Build history of the part. All positions in model axes, mm. Face numbers are marked on the shaded views. A direction names the side the tool comes from. Give positions to 0.01 mm unless a question says otherwise; leave off trailing zeros. Loops run counter-clockwise (first coordinate to the right, second up) from the corner with the lowest first, then second, coordinate; pieces in that order, holes last. Notation, with made-up numbers: M 65.25,50.25 L 72.25,50.25 A34 cw 72.25,89.25 Z; hole C -29.75,6 d4. An arc over 180 degrees is marked long. Put each result on its own line as item: value.
```python
from build123d import *

# Parameters (mm, degrees)
F1_DEPTH      = 19.05
F2_R          = 8.200531
F3_DEPTH      = 38.1
F3_DEPTH_BACK = 25.4
F5_DEPTH      = 38.1


with BuildPart() as f1:
    # F0 (on Front) → F1 (new body, symmetric)
    with BuildSketch(Plane.XZ):
        with BuildLine():
            Line((-32.141831, 33.15654), (-26.644221, 0))
            Line((-26.644221, 0), (-32.141831, -48.038937))
            Line((-32.141831, -48.038937), (-37.479226, -82.203552))
            Line((-37.479226, -82.203552), (-48.503112, -88.604517))
            Line((-48.503112, -88.604517), (-48.503112, -100.208476))
            Line((-48.503112, -100.208476), (-13.84278, -100.208476))
            Line((-13.84278, -100.208476), (0, -20.61474))
            Line((0, -20.61474), (0, 124.924347))
            ThreePointArc((0, 124.924347), (-20.562864, 109.037436), (-6.345349, 87.28686))
            Line((-6.345349, 87.28686), (-18.186359, 69.102459))
            Line((-18.186359, 69.102459), (-43.982837, 61.913271))
            Line((-43.982837, 61.913271), (-71.473219, 31.58654))
            Line((-71.473219, 31.58654), (-64.171686, 6.32793))
            Line((-64.171686, 6.32793), (-53.286485, 9.474526))
            Line((-53.286485, 9.474526), (-57.54343, 24.200819))
            Line((-57.54343, 24.200819), (-43.137055, 42.037293))
            Line((-43.137055, 42.037293), (-32.141831, 33.15654))
        make_face()
        with BuildLine():
            Line((0, 124.924347), (0, -20.61474))
            Line((0, -20.61474), (13.84278, -100.208476))
            Line((13.84278, -100.208476), (48.503112, -100.208476))
            Line((48.503112, -100.208476), (48.503112, -88.604517))
            Line((48.503112, -88.604517), (37.479226, -82.203552))
            Line((37.479226, -82.203552), (32.141831, -48.038937))
            Line((32.141831, -48.038937), (26.644221, 0))
            Line((26.644221, 0), (32.141831, 33.15654))
            Line((32.141831, 33.15654), (43.137055, 42.037293))
            Line((43.137055, 42.037293), (57.54343, 24.200819))
            Line((57.54343, 24.200819), (53.286485, 9.474526))
            Line((53.286485, 9.474526), (64.171686, 6.32793))
            Line((64.171686, 6.32793), (71.473219, 31.58654))
            Line((71.473219, 31.58654), (43.982837, 61.913271))
            Line((43.982837, 61.913271), (18.186359, 69.102459))
            Line((18.186359, 69.102459), (6.345349, 87.28686))
            ThreePointArc((6.345349, 87.28686), (20.562864, 109.037436), (0, 124.924347))
        make_face()
    extrude(amount=F1_DEPTH, both=True)

    # F2 (on face) → F3 (cut, two sides)
    with BuildSketch(Plane.XZ.offset(19.05)) as f3_sk:
        with Locations((-10.217502, 107.796535)):
            Circle(F2_R)
        with Locations((10.217502, 107.796535)):
            Circle(F2_R)
    extrude(amount=-F3_DEPTH, mode=Mode.SUBTRACT)
    extrude(f3_sk.sketch, amount=-F3_DEPTH_BACK, mode=Mode.SUBTRACT)

    # F4 (on face) → F5 (join, through all)
    with BuildSketch(Plane(origin=(0, 19.05, 0), x_dir=(-1, 0, 0), z_dir=(0, 1, 0))):
        with BuildLine():
            ThreePointArc((-6.158323, 124.468817), (-8.54694, 126.271077), (-9.095944, 129.212543))
            ThreePointArc((-9.095944, 129.212543), (-10.942716, 126.29527), (-10.440769, 122.879263))
            ThreePointArc((-10.440769, 122.879263), (-8.347127, 123.802228), (-6.158323, 124.468817))
        make_face()
        with BuildLine():
            ThreePointArc((-16.136752, 118.410561), (-15.235, 119.378746), (-14.268527, 120.282334))
            ThreePointArc((-14.268527, 120.282334), (-15.496071, 121.489871), (-15.748994, 123.193115))
            ThreePointArc((-15.748994, 123.193115), (-16.894778, 120.879016), (-16.136752, 118.410561))
        make_face()
        with BuildLine():
            ThreePointArc((9.095944, 129.212543), (8.54694, 126.271077), (6.158323, 124.468817))
            ThreePointArc((6.158323, 124.468817), (8.347127, 123.802228), (10.440769, 122.879263))
            ThreePointArc((10.440769, 122.879263), (10.942716, 126.29527), (9.095944, 129.212543))
        make_face()
        with BuildLine():
            ThreePointArc((15.748994, 123.193115), (15.496071, 121.489871), (14.268527, 120.282334))
            ThreePointArc((14.268527, 120.282334), (15.235, 119.378746), (16.136752, 118.410561))
            ThreePointArc((16.136752, 118.410561), (16.894778, 120.879016), (15.748994, 123.193115))
        make_face()
    extrude(amount=-F5_DEPTH)


solid = f1.part
```
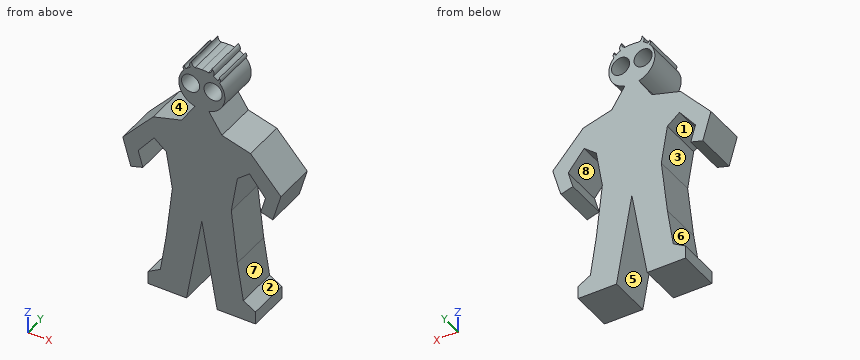
Q1. Mould opens along X. For the marked faces 1, 2, 3 and 4 say: pulls with the +X half, pulls with the -X half, needs draft (parallel to the pull), parting line crosses it, or undercut.
Here are the results:
face 1: undercut
face 2: pulls with the +X half
face 3: undercut
face 4: pulls with the -X half
Q2. Slice it at C-C (y = 14.5). State how many separate pieces and enclosed holes the cut face has, and give its area (3 significant figures).
Here are the results:
separate pieces: 1
enclosed holes: 2
area: 13,300 mm²
Q3. Probe line 1 (X direction, y = 1, z = 28.5); line 2 (Z direction, x = 45.5, y = 4); line 3 (X direction, y = -17, z = 11). List the from-to ranges inside material, lowest first. Write a range as from..to.
Here are the results:
line 1: -70.58..-54.07, -31.37..31.37, 54.07..70.58
line 2: -100.21..-86.86, 39.11..60.24
line 3: -65.52..-53.73, -28.47..28.47, 53.73..65.52
Q4. Slice it at B-B (z = -78.5). List the corners of the cut face in (x, y), and give its area (3 significant figures).
Here are the results:
outline: M -36.9,-19.05 L -10.07,-19.05 L -10.07,19.05 L -36.9,19.05 Z; M 10.07,-19.05 L 36.9,-19.05 L 36.9,19.05 L 10.07,19.05 Z
area: 2,040 mm²
Q5. Slice it at A-A (z = 105). List the corners of the cut face in (x, y), and give its area (3 significant figures).
Here are the results:
outline: M -20.81,-19.05 L -17.93,-19.05 L -17.93,19.05 L -20.81,19.05 Z; M -2.51,-19.05 L 2.51,-19.05 L 2.51,19.05 L -2.51,19.05 Z; M 17.93,-19.05 L 20.81,-19.05 L 20.81,19.05 L 17.93,19.05 Z
area: 411 mm²
Q6. Slice it at D-D (z = -25). List the corners of the cut face in (x, y).
Here are the results:
outline: M -29.51,-19.05 L -0.76,-19.05 L -0.76,19.05 L -29.51,19.05 Z; M 0.76,-19.05 L 29.51,-19.05 L 29.51,19.05 L 0.76,19.05 Z
Q7. Tool access for the marked faces 5, 6, 7 and 8: list every direction of +Z, -Z, +X, -X, +Y, -Y with a clear straight run to the whole face (end or side of a thin tool).
Here are the results:
face 5: -Z, +Y, -Y
face 6: -X, +Y, -Y
face 7: +X, +Y, -Y
face 8: +Y, -Y
Q8. Drop flat-ended pins along their axis: pin 1 Ø10 at (y, z) = (7.5, 11) entering from -X; pin 2 Ø3 at (y, z) = (12, -41) entering from +X; pin 3 Ø5 at (y, z) = (-1, 98.5) entering from +X. Give the stop position or say it passes through.
Here are the results:
pin 1: x = -66.97
pin 2: x = 31.51
pin 3: x = 20.2
